For this review, take the finished solid that the model builds, in its own axes (mm). A direction names the side the tool comes from. Round coordinates to 2 decimals unless told otherwise and drop trailing zeros. Order: outer loops, then holes, each group sorted by start corner. A loop starts at its lowest first (then second) coordinate and runs counter-clockwise, first axis right, second up.
from build123d import *

# Parameters (mm, degrees)
SKETCH1_W          = 266
SKETCH1_H          = 25.5
BASE_FLANGE1_DEPTH = 1
HEM1_START         = -133
HEM1_DEPTH         = 266
HEM1_2_DEPTH       = 266
CUT_EXTRUDE1_START = -134.703262862
SKETCH8_W          = 14
SKETCH8_H          = 6
CUT_EXTRUDE1_DEPTH = 259.406525724
LPATTERN1_COUNT    = 11
LPATTERN1_PITCH    = 28
CHAMFER1_SIZE      = 0.5
SKETCH9_R          = 2
CUT_EXTRUDE2_DEPTH = 10
LPATTERN2_COUNT    = 5
LPATTERN2_PITCH    = 60
CHAMFER2_SIZE      = 1


# Read off the part's stored shape, not the designer's step: Hem1
# Sheet-metal steps are written as plain solids
with BuildPart() as part:
    # Sketch1 → Base-Flange1 (new body)
    with BuildSketch(Plane(origin=(0, 0, 0), x_dir=(1, 0, 0), z_dir=(0, 1, 0))):
        Rectangle(SKETCH1_W, SKETCH1_H)
    extrude(amount=-BASE_FLANGE1_DEPTH)

    # Hem1 outline → Hem1 (cut)
    with BuildSketch(Plane.YZ.offset(HEM1_START)):
        with BuildLine():
            Line((0, -12.75), (0, -11.986067977))
            ThreePointArc((0, -11.986067977), (-0.738612788, -10.974744871), (-1, -9.75))
            Line((-1, -9.75), (-1, -12.75))
            Line((-1, -12.75), (0, -12.75))
        make_face()
    extrude(amount=HEM1_DEPTH, mode=Mode.SUBTRACT)

    # Hem1 2 outline → Hem1 2 (add)
    with BuildSketch(Plane.YZ.offset(HEM1_START)):
        with BuildLine():
            Line((0.732145215, -7.031076639), (1.154763477, -7.937384426))
            ThreePointArc((1.154763477, -7.937384426), (3.686782892, -10.824599218), (0, -9.75))
            Line((0, -9.75), (0, -11.986067977))
            ThreePointArc((0, -11.986067977), (4.967777538, -10.18851623), (0.732145215, -7.031076639))
        make_face()
    extrude(amount=HEM1_2_DEPTH)

    # Sketch8 → Cut-Extrude1 (cut)
    with BuildSketch(Plane(origin=(0, 0, 0), x_dir=(1, 0, 0), z_dir=(0, 1, 0)).offset(CUT_EXTRUDE1_START)):
        with Locations((112, 9.75)):
            Rectangle(SKETCH8_W, SKETCH8_H)
    cut_extrude1 = extrude(amount=CUT_EXTRUDE1_DEPTH, mode=Mode.SUBTRACT)

    # LPattern1: Cut-Extrude1 ×11
    with Locations(*[(-i * LPATTERN1_PITCH, 0, 0) for i in range(1, LPATTERN1_COUNT)]):
        add(cut_extrude1, mode=Mode.SUBTRACT)

    # Chamfer1
    chamfer1_edges = [part.edges().sort_by_distance(p)[0] for p in [
        (-133, 0, 1.5),
        (133, 3.686782892, -10.824599218),
        (-133, 3.686782892, -10.824599218),
        (-133, 0, 1.5),
        (0, 0, 12.75),
        (133, 0, 1.5),
    ]]
    chamfer(chamfer1_edges, length=CHAMFER1_SIZE)

    # Sketch9 → Cut-Extrude2 (cut)
    with BuildSketch(Plane(origin=(0, 0, 0), x_dir=(1, 0, 0), z_dir=(0, 1, 0))):
        with Locations(Location((-120, -1.25, 0), (0, 0, 270))):
            Circle(SKETCH9_R)
    cut_extrude2 = extrude(amount=-CUT_EXTRUDE2_DEPTH, mode=Mode.SUBTRACT)

    # LPattern2: Cut-Extrude2 ×5
    with Locations(*[(i * LPATTERN2_PITCH, 0, 0) for i in range(1, LPATTERN2_COUNT)]):
        add(cut_extrude2, mode=Mode.SUBTRACT)

    # Chamfer2
    chamfer2_edges = [part.edges().sort_by_distance(p)[0] for p in [
        (-120, 0, -0.75),
        (-60, 0, -0.75),
        (0, 0, -0.75),
        (60, 0, -0.75),
        (120, 0, -0.75),
    ]]
    chamfer(chamfer2_edges, length=CHAMFER2_SIZE - 0.0001)  # a hair under: the kernel refuses the full size


solid = part.part
(1) Wall thickness on L1, parallel to X at y = -0.95, z = 1.25; L2, parallel to Z at x = 68.5, y = 2; L3, parallel to Y at x = 46.25, z = -9.75: over which ranges is each line inside the solid? List them lowest first.
(2) Clearance check with flat-ended pins moving along their axes: P1, Ø0.5, axis at x = -1.5, y = -0.5, coming from the -Z side; P2, Ø4, axis at x = 42, z = 1, coming from the +Y side; P3, Ø1, axis at x = 92, y = 1, coming from the +Z side. State where each tip first meets the part, or that it passes through.
(3) Add section B-B on z = -4. Give the boundary of the cut face in (x, y).
(4) Add section C-C on x = 16.5. Give the boundary of the cut face in (y, z).
(5) Draft analysis for pull direction X (two halves, no side actions). For faces 1 (the face through (-1.9, 0, -1.3)), 2 (the face through (-132.64, 3.76, -10.97)), 3 (the face through (21, 1.3, -7.7)), state which applies: pulls with the +X half, pulls with the -X half, needs draft (parallel to the pull), parting line crosses it, or undercut.
(6) Tool access review of faces 4 (the face through (-133, -0.7, -3.7)), 5 (the face through (-49, 1.3, -7.7)): name each direction out of +Z, -Z, +X, -X, +Y, -Y from which nothing blocks a thin tool from reaching the whole face with its end or side.
(7) Add section A-A on x = 54. Give the boundary of the cut face in (y, z).
Here are the results:
1. L1: x = -133 to -122.05, -117.95 to -62.05, -57.95 to -2.05, 2.05 to 57.95, 62.05 to 117.95, 122.05 to 133
1. L2: z = -12.75 to -11.75, -7.75 to -6.75
1. L3: y = -1 to 0, 4 to 5
2. P1: stops at z = -6.75
2. P2: stops at y = 0
2. P3: stops at z = -6.79
3. outline: (-133, -1) - (133, -1) - (133, -0.5) - (132.5, 0) - (-132.5, 0) - (-133, -0.5) - close
4. outline: (-1, -9.75) arc R3 ccw (long way) to (0.73, -7.03) - (1.15, -7.94) arc R2 cw (long way) to (0, -9.75) - (0, 12.25) - (-0.5, 12.75) - (-1, 12.75) - close
5. face 1: needs draft
5. face 2: pulls with the -X half
5. face 3: undercut
6. face 4: +Z, -Z, -X, +Y, -Y
6. face 5: -Z, +Y, -Y
7. outline: (-1, -6.75) - (0, -6.75) - (0, 12.25) - (-0.5, 12.75) - (-1, 12.75) - close
